from build123d import *

# Parameters (mm, degrees)
SKETCH1_R           = 1.6
SKETCH1_R_2         = 2.5
BOSS_EXTRUDE1_DEPTH = 1.57


with BuildPart() as part:
    # Sketch1 → Boss-Extrude1 (new body)
    with BuildSketch(Plane(origin=(0, 1.57, 0), x_dir=(1, 0, 0), z_dir=(0, 1, 0))):
        with BuildLine():
            Line((0, -5), (16.5, -5))
            ThreePointArc((16.5, -5), (21.224261413, -1.637484075), (19.594361133, 3.927458361))
            Line((19.594361133, 3.927458361), (3.094361133, 16.927458361))
            ThreePointArc((3.094361133, 16.927458361), (-2.182681188, 17.498433375), (-5, 13))
            Line((-5, 13), (-5, 0))
            ThreePointArc((-5, 0), (-3.535533906, -3.535533906), (0, -5))
        make_face()
        with Locations((0, 13)):
            Circle(SKETCH1_R, mode=Mode.SUBTRACT)
        with Locations((16.5, 0)):
            Circle(SKETCH1_R, mode=Mode.SUBTRACT)
        Circle(SKETCH1_R_2, mode=Mode.SUBTRACT)
    extrude(amount=-BOSS_EXTRUDE1_DEPTH)


solid = part.part
Check sheet for the modelled part. Datum: model origin and axes. Units: mm. Round coordinates to 2 decimals unless told otherwise and drop trailing zeros. Loops run counter-clockwise (first coordinate to the right, second up) from the corner with the lowest first, then second, coordinate; pieces in that order, holes last.
1. Mould release check, pull along X, two halves, no side actions. Record for faces 1 (the flat face through (5, 0, -4)), 2 (the cylindrical face through (-0.208, 0.796, -14.586)), 3 (the cylindrical face through (-2.112, 0.796, -17.532)): released by +X, released by -X, zero draft, split by the parting line, or undercut.
2. Sectioned sample at C-C on z = 3.75. Record the boundary of the cut face in (x, y).
3. Sectioned sample at B-B on x = 5.25. Record the boundary of the cut face in (y, z).
4. Gauge pin test, flat end, axial feed: pin 1 Ø4.5 at (x, z) = (0, 0) entering from +Y. Record the tip position at first contact, or that the pin passes through.
5. Sectioned sample at A-A on y = 1.05. Record the boundary of the cut face in (x, z).
6. Scan lines: probe 1 along X at (y, z) = (1.1, 0); probe 2 along X at (y, z) = (0.2, -0.5); probe 3 along X at (y, z) = (0.1, -1.75). Record each from-to range of solid material in increasing order.
Recorded:
1. face 1: zero draft
1. face 2: undercut
1. face 3: split by the parting line
2. outline: (-3.31, 0) - (19.81, 0) - (19.81, 1.57) - (-3.31, 1.57) - close
3. outline: (0, -15.23) - (1.57, -15.23) - (1.57, 5) - (0, 5) - close
4. pin 1: passes through
5. outline: (-5, -13) arc R5 ccw to (3.09, -16.93) - (19.59, -3.93) arc R5 ccw to (16.5, 5) - (0, 5) arc R5 ccw to (-5, 0) - close; hole circle Ø5 at (0, 0); hole circle Ø3.2 at (0, -13); hole circle Ø3.2 at (16.5, 0)
6. probe 1: x = -5 to -2.5, 2.5 to 14.9, 18.1 to 21.5
6. probe 2: x = -5 to -2.45, 2.45 to 14.98, 18.02 to 21.47
6. probe 3: x = -5 to -1.79, 1.79 to 21.18
